Input: dimensioned drawing with shaded views. Units: mm. Origin: part minimum x, y, z. A direction names the side the tool comes from. Give positions to 0.01 mm unless a question says otherwise; leave off trailing zeros. Loops run counter-clockwise (first coordinate to the right, second up) from the corner with the lowest first, then second, coordinate; pieces in that order, holes last.
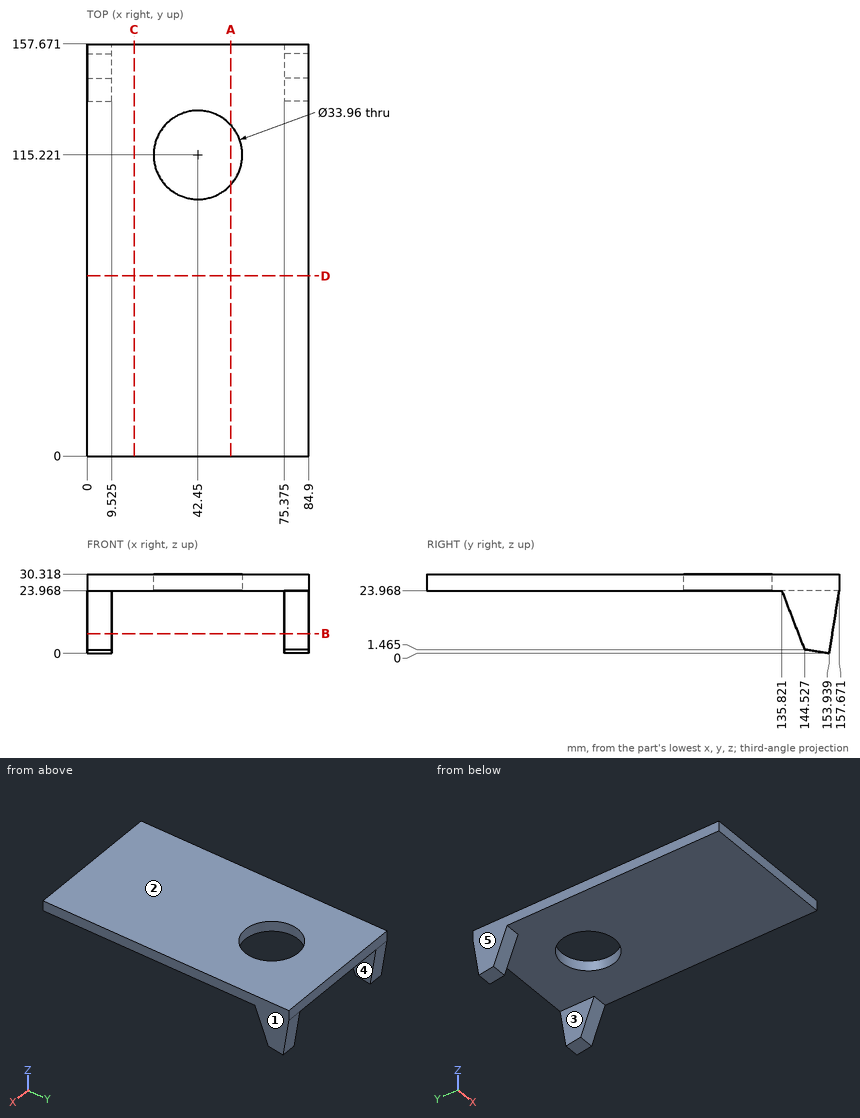
Item 1: Section query B-B on z = 7.5. Return loops of the section in (x, y) (1 decimal), plus the area to 3 significant figures.
Values follow:
outline: (0, 142.2) - (9.5, 142.2) - (9.5, 155.1) - (0, 155.1) - close; (75.4, 142.2) - (84.9, 142.2) - (84.9, 155.1) - (75.4, 155.1) - close
area: 246 mm2
Item 2: Set-up query: the marked faces 4 and 5. Return all of +Z, -Z, +X, -X, +Y, -Y with unobstructed straight access to the full face (end or side cutting, diameter ignored); none if empty.
Values follow:
face 4: -Z, +Y, -Y
face 5: +Z, -Z, -X, +Y, -Y
Item 3: Draft query along X for the marked faces 1, 2 and 3. Return one class per face: +X half, -X half, draft (parallel to the pull), parting line (faces both ways), or undercut.
Values follow:
face 1: +X half
face 2: draft
face 3: undercut
Item 4: Section query C-C on x = 18. Return loops of the section in (y, z), plus the area to 3 significant figures.
Values follow:
outline: (0, 23.97) - (157.67, 23.97) - (157.67, 30.32) - (0, 30.32) - close
area: 1,000 mm2
Item 5: Section query D-D on y = 69. Return loops of the section in (x, z), plus the area to 3 significant figures.
Values follow:
outline: (0, 23.97) - (84.9, 23.97) - (84.9, 30.32) - (0, 30.32) - close
area: 539 mm2
Item 6: Ray query, probe 1 along Z at (x, y) = (60, 69); probe 2 along Y at (x, z) = (36, 27) (1 decimal); probe 3 along Y at (x, z) = (7, 14). Return the intervals inside material, ascending.
Values follow:
probe 1: z = 23.97 to 30.32
probe 2: y = 0 to 99.5, 130.9 to 157.7
probe 3: y = 139.68 to 156.12
Item 7: Section query A-A on x = 55. Return loops of the section in (y, z).
Values follow:
outline: (0, 23.97) - (103.78, 23.97) - (103.78, 30.32) - (0, 30.32) - close; (126.66, 23.97) - (157.67, 23.97) - (157.67, 30.32) - (126.66, 30.32) - close
Item 8: Pin query (flat end, axial travel): pin 1 (2 mm diameter, centred on x = 30.5, y = 20.5, fed in from -Z). Return the tip coordinate at first contact, or that it passes through.
Values follow:
pin 1: stops at z = 23.97
